Verification items for the finished model (mm, model axes). Face numbers are marked on the shaded views. Coordinates: 2 decimals unless noted, no trailing zeros. Write each loop counter-clockwise with the first axis right and the second up, starting at its lowest first coordinate (ties: lowest second). Pieces come first, ordered by that corner, then holes. Notation, with made-up numbers: (44.25, 81.25) -> (83.25, 81.25) arc R18 cw to (83.25, 95.25) -> close; hole circle Ø7 at (-37, 8.25). An arc over 180 degrees is marked (long way). Answer in a Markdown table with one row per item.
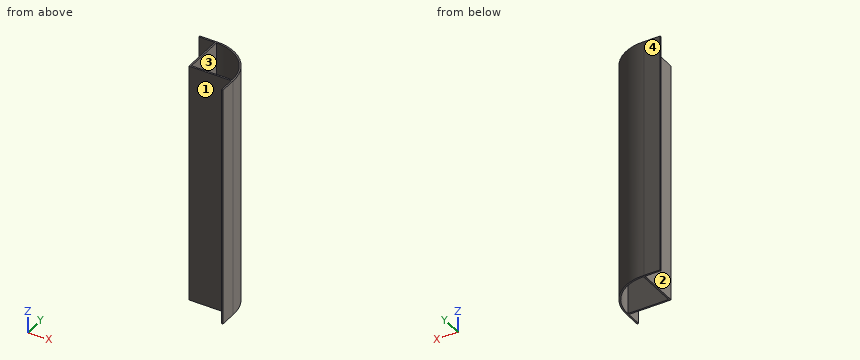
```python
from build123d import *

# Parameters (mm, degrees)
CROQUIS1_W              = 10
CROQUIS1_H              = 1
CROQUIS1_W_2            = 1
CROQUIS1_H_2            = 10
SALIENTE_EXTRUIR1_DEPTH = 75


with BuildPart() as part:
    # Croquis1 → Saliente-Extruir1 (new body, symmetric)
    with BuildSketch(Plane.XY):
        with BuildLine():
            ThreePointArc((-13.7, 13.681053808), (5.967619023, 5.967619023), (13.681053808, -13.7))
            Line((13.681053808, -13.7), (-13.7, -13.7))
            Line((-13.7, -13.7), (-13.7, 13.681053808))
        make_face()
        with BuildLine():
            Line((-12.7, -12.7), (-12.7, 12.7))
            ThreePointArc((-12.7, 12.7), (5.260512242, 5.260512242), (12.7, -12.7))
            Line((12.7, -12.7), (-12.7, -12.7))
        make_face(mode=Mode.SUBTRACT)
        with Locations((-18.7, 13.181053808)):
            Rectangle(CROQUIS1_W, CROQUIS1_H)
        with Locations((13.181053808, -18.7)):
            Rectangle(CROQUIS1_W_2, CROQUIS1_H_2)
    extrude(amount=SALIENTE_EXTRUIR1_DEPTH, both=True)


solid = part.part
```
1. Sectioned sample at C-C, the plane x = -4. Record the cut outline in (y, z).
Findings below:
| item | result |
|---|---|
| outline | (-13.7, -75) -> (-12.7, -75) -> (-12.7, 75) -> (-13.7, 75) -> close; (11.16, -75) -> (12.23, -75) -> (12.23, 75) -> (11.16, 75) -> close |
2. Sectioned sample at A-A, the plane z = 13.5. Record the cut outline in (x, y).
Findings below:
| item | result |
|---|---|
| outline | (-23.7, 12.68) -> (-13.7, 12.68) -> (-13.7, -13.7) -> (12.68, -13.7) -> (12.68, -23.7) -> (13.68, -23.7) -> (13.68, -13.7) arc R26.4 ccw to (-13.7, 13.68) -> (-23.7, 13.68) -> close; hole (-12.7, -12.7) -> (12.7, -12.7) arc R25.4 ccw to (-12.7, 12.7) -> close |
3. Sectioned sample at B-B, the plane y = 10. Record the cut outline in (x, z).
Findings below:
| item | result |
|---|---|
| outline | (-13.7, -75) -> (-12.7, -75) -> (-12.7, 75) -> (-13.7, 75) -> close; (-1.3, -75) -> (0.78, -75) -> (0.78, 75) -> (-1.3, 75) -> close |
4. Go/stop test with flat-tipped pins: pin 1 (3 mm diameter, centred on y = -15, z = -50, fed in from -X); pin 2 (3 mm diameter, centred on x = -16, z = -17, fed in from +Y); pin 3 (8 mm diameter, centred on x = -4.5, z = 14.5, fed in from -Y). Record where each tip stops, or that it passes through.
Findings below:
| item | result |
|---|---|
| pin 1 | stops at x = -13.7 |
| pin 2 | stops at y = 13.68 |
| pin 3 | stops at y = -13.7 |
5. Material ranges on probe 1 along X at (y, z) = (-12, 48); probe 2 along Y at (x, z) = (-21.5, 31); probe 3 along X at (y, z) = (-11, -67.5), recorded low to high. Write a range as from..to.
Findings below:
| item | result |
|---|---|
| probe 1 | x = -13.7..-12.7, 12.69..13.69 |
| probe 2 | y = 12.68..13.68 |
| probe 3 | x = -13.7..-12.7, 12.64..13.65 |
6. Sectioned sample at D-D, the plane x = -15. Record the cut outline in (y, z).
Findings below:
| item | result |
|---|---|
| outline | (12.68, -75) -> (13.68, -75) -> (13.68, 75) -> (12.68, 75) -> close |
7. Release check for a two-part mould opening along Y. For the marked faces 1, 2, 3 and 4 record: released by +Y, released by -Y, zero draft, split by the parting line, or undercut.
Findings below:
| item | result |
|---|---|
| face 1 | released by -Y |
| face 2 | zero draft |
| face 3 | undercut |
| face 4 | released by +Y |
